Autodesk Inventor part; units mm, degrees
ref_plane "YZ Plane" through (0, 0, 0) normal (1, 0, 0) x (0, 1, 0)
ref_plane "XZ Plane" through (0, 0, 0) normal (0, 1, 0) x (-1, 0, 0)
ref_plane "XY Plane" through (0, 0, 0) normal (0, 0, 1) x (1, 0, 0)
sketch "Sketch1" plane through (0, 0, 0) normal (0, 0, 1) x (1, 0, 0)
  line L0 (0, -252.5291) -> (0, 252.5291) construction
  line L1 (-273, 0) -> (273, 0) construction
  line L2 (-195, 100) -> (195, 100)
  line L3 (195, 100) -> (195, -100)
  line L4 (195, -100) -> (-195, -100)
  line L5 (-195, -100) -> (-195, 100)
  line L6 (-178.1654, -28.1654) -> (-178.1654, 28.1654) construction
  line L7 (-178.1654, 28.1654) -> (178.1654, 28.1654) construction
  line L8 (178.1654, 28.1654) -> (178.1654, -28.1654) construction
  line L9 (178.1654, -28.1654) -> (-178.1654, -28.1654) construction
  circle A0 centre (0, 0) radius 180.3779 construction
  line L10 (-175, 25) -> (-175, -25) construction
  line L11 (-175, -25) -> (175, -25) construction
  line L12 (175, -25) -> (175, 25) construction
  line L13 (175, 25) -> (-175, 25) construction
  circle A1 centre (-175, 0) radius 6 construction
  point P0 (175, 0)
  point P1 (0, 25)
  point P2 (0, -25)
  dimension "d0" = 390
  dimension "d1" = 200
  dimension "d5" = 350
  dimension "d6" = 360.7559
  dimension "d14" = 350
  dimension "d15" = 12
  dimension "d54" = 353.5534
  dimension "d104" = 350
  dimension "d105" = 50
extrude "Extrusion1" add sketch "Sketch1" along normal blind 10
sketch "Sketch2" plane through (0, 0, 10) normal (0, 0, 1) x (1, 0, 0)
  point P0 (0, 0)
  point P1 (-175, -25)
  point P2 (-175, 25)
  point P3 (175, 25)
  point P4 (175, -25)
  point P5 (-175, 0)
  point P6 (175, 0)
  point P7 (0, 25)
  point P8 (0, -25)
hole "Hole1" at (-175, -25, 10) at (175, 25, 10) at (-175, 25, 10) at (175, -25, 10) at (0, 25, 10) at (0, -25, 10) direction (0, 0, -1) diameter 4.917 end through all
hole "Hole2" at (-175, 0, 10) at (175, 0, 10) direction (0, 0, -1) diameter 6.5 end through all counterbore diameter 16.5 counterbore depth 2
sketch "Sketch3" plane through (0, 0, 10) normal (0, 0, 1) x (1, 0, 0)
  line L0 (195, 100) -> (-195, 100) construction
  line L1 (-195, -100) -> (195, -100) construction
  line L2 (-195, 100) -> (-195, -100) construction
  line L3 (-273, 0) -> (273, 0) construction
  line L4 (0, -140) -> (0, 140) construction
  line L5 (195, -100) -> (195, 100) construction
  line L6 (-180, 90) -> (180, 90) construction
  line L7 (180, 90) -> (180, -90) construction
  line L8 (180, -90) -> (-180, -90) construction
  line L9 (-180, -90) -> (-180, 90) construction
  point P0 (0, 0)
  point P1 (-170, 80)
  point P2 (-150, 80)
  point P3 (-150, 80)
  point P4 (-130, 80)
  point P5 (-110, 80)
  point P6 (-90, 80)
  point P7 (-70, 80)
  point P8 (-50, 80)
  point P9 (-30, 80)
  point P10 (-10, 80)
  point P11 (10, 80)
  point P12 (30, 80)
  point P13 (50, 80)
  point P14 (70, 80)
  point P15 (90, 80)
  point P16 (110, 80)
  point P17 (130, 80)
  point P18 (150, 80)
  point P19 (170, 80)
  point P20 (-170, 60)
  point P21 (-150, 60)
  point P22 (-130, 60)
  point P23 (-110, 60)
  point P24 (-90, 60)
  point P25 (-70, 60)
  point P26 (-50, 60)
  point P27 (-30, 60)
  point P28 (-10, 60)
  point P29 (10, 60)
  point P30 (30, 60)
  point P31 (50, 60)
  point P32 (70, 60)
  point P33 (90, 60)
  point P34 (110, 60)
  point P35 (130, 60)
  point P36 (150, 60)
  point P37 (170, 60)
  point P38 (-170, 40)
  point P39 (-150, 40)
  point P40 (-130, 40)
  point P41 (-110, 40)
  point P42 (-90, 40)
  point P43 (-70, 40)
  point P44 (-50, 40)
  point P45 (-30, 40)
  point P46 (-10, 40)
  point P47 (10, 40)
  point P48 (30, 40)
  point P49 (50, 40)
  point P50 (70, 40)
  point P51 (90, 40)
  point P52 (110, 40)
  point P53 (130, 40)
  point P54 (150, 40)
  point P55 (170, 40)
  point P56 (-170, 20)
  point P57 (-150, 20)
  point P58 (-130, 20)
  point P59 (-110, 20)
  point P60 (-90, 20)
  point P61 (-70, 20)
  point P62 (-50, 20)
  point P63 (-30, 20)
  point P64 (-10, 20)
  point P65 (10, 20)
  point P66 (30, 20)
  point P67 (50, 20)
  point P68 (70, 20)
  point P69 (90, 20)
  point P70 (110, 20)
  point P71 (130, 20)
  point P72 (150, 20)
  point P73 (170, 20)
  point P74 (-170, 0)
  point P75 (-150, 0)
  point P76 (-130, 0)
  point P77 (-110, 0)
  point P78 (-90, 0)
  point P79 (-70, 0)
  point P80 (-50, 0)
  point P81 (-30, 0)
  point P82 (-10, 0)
  point P83 (10, 0)
  point P84 (30, 0)
  point P85 (50, 0)
  point P86 (70, 0)
  point P87 (90, 0)
  point P88 (110, 0)
  point P89 (130, 0)
  point P90 (150, 0)
  point P91 (170, 0)
  point P92 (-170, -20)
  point P93 (-150, -20)
  point P94 (-130, -20)
  point P95 (-110, -20)
  point P96 (-90, -20)
  point P97 (-70, -20)
  point P98 (-50, -20)
  point P99 (-30, -20)
  point P100 (-10, -20)
  point P101 (10, -20)
  point P102 (30, -20)
  point P103 (50, -20)
  point P104 (70, -20)
  point P105 (90, -20)
  point P106 (110, -20)
  point P107 (130, -20)
  point P108 (150, -20)
  point P109 (170, -20)
  point P110 (-170, -40)
  point P111 (-150, -40)
  point P112 (-130, -40)
  point P113 (-110, -40)
  point P114 (-90, -40)
  point P115 (-70, -40)
  point P116 (-50, -40)
  point P117 (-30, -40)
  point P118 (-10, -40)
  point P119 (10, -40)
  point P120 (30, -40)
  point P121 (50, -40)
  point P122 (70, -40)
  point P123 (90, -40)
  point P124 (110, -40)
  point P125 (130, -40)
  point P126 (150, -40)
  point P127 (170, -40)
  point P128 (-170, -60)
  point P129 (-150, -60)
  point P130 (-130, -60)
  point P131 (-110, -60)
  point P132 (-90, -60)
  point P133 (-70, -60)
  point P134 (-50, -60)
  point P135 (-30, -60)
  point P136 (-10, -60)
  point P137 (10, -60)
  point P138 (30, -60)
  point P139 (50, -60)
  point P140 (70, -60)
  point P141 (90, -60)
  point P142 (110, -60)
  point P143 (130, -60)
  point P144 (150, -60)
  point P145 (170, -60)
  point P146 (-170, -80)
  point P147 (-150, -80)
  point P148 (-130, -80)
  point P149 (-110, -80)
  point P150 (-90, -80)
  point P151 (-70, -80)
  point P152 (-50, -80)
  point P153 (-30, -80)
  point P154 (-10, -80)
  point P155 (10, -80)
  point P156 (30, -80)
  point P157 (50, -80)
  point P158 (70, -80)
  point P159 (90, -80)
  point P160 (110, -80)
  point P161 (130, -80)
  point P162 (150, -80)
  point P163 (170, -80)
  dimension "d25" = 10
  dimension "d26" = 360
  dimension "d27" = 180
  dimension "d28" = 10
  dimension "d29" = 10
  dimension "d30" = 20
  dimension "d33" = 20
  dimension "d36" = 20
  dimension "d39" = 15
hole "Hole3" [suppressed]
hole "Hole4" at (0, 0, 10) direction (0, 0, -1) diameter 11 end through all
sketch "Sketch4" plane through (0, 0, 0) normal (0, 0, -1) x (-1, 0, 0)
  circle A0 centre (175, 0) radius 3.25 construction
  circle A1 centre (-175, 0) radius 3.25 construction
  line L0 (195, -100) -> (-195, -100) construction
  line L1 (187.5, -100) -> (187.5, 100) construction
  line L2 (-195, 100) -> (195, 100) construction
  line L3 (273, 0) -> (-273, 0) construction
  line L4 (0, -140) -> (0, 140) construction
  line L5 (195, 100) -> (195, -100) construction
  point P0 (0, 0)
  point P1 (187.5, -90)
  point P2 (187.5, 90)
  point P3 (187.5, 0)
  point P4 (-187.5, -90)
  point P5 (-187.5, 90)
  point P6 (-187.5, 0)
  dimension "d62" = 180
  dimension "d63" = 7.5
hole "Hole5" at (-175, 0, 0) at (175, 0, 0) direction (0, 0, 1) diameter 6.5 end through all countersink diameter 14.5 countersink angle 90
hole "Hole6" at (-187.5, -90, 0) at (-187.5, 90, 0) at (-187.5, 0, 0) at (187.5, -90, 0) at (187.5, 0, 0) at (187.5, 90, 0) direction (0, 0, 1) diameter 3.242 end through all
sketch "Sketch10" plane through (-195, -100, 0) normal (0, -1, 0) x (1, 0, 0)
  line L0 (0, 0) -> (0, 10) construction
  line L1 (0, 6) -> (390, 6) construction
  line L2 (390, 0) -> (390, 10) construction
  line L3 (195, -2) -> (195, 12) construction
  line L4 (0, 10) -> (390, 10) construction
  line L5 (0, 0) -> (390, 0) construction
  point P0 (195, 0)
  point P1 (60, 6)
  point P2 (330, 6)
  dimension "d95" = 270
  dimension "d103" = 6
hole "Hole10" at (-135, -100, 6) at (135, -100, 6) direction (0, 1, 0) diameter 3.242 depth 15 tip angle 118
fillet "Fillet1" radius 2 4 edges at (-195, -100, 5) (195, -100, 5) (-195, 100, 5) (195, 100, 5)
properties part number "DLT-01-231B" material "Acrílico TP"
Source: CAD feature listing. Evaluate the final solid. Frame: model axes, mm. A direction names the side the tool comes from. Coordinates: 2 decimals unless noted, no trailing zeros. Answer as a JSON object with one key per item and string values.
Q1. Draft query along Y for faces 3 (the conical face through (-178.105, 1.615, 3.75)), 4 (the flat face through (-3, -21, 10)), 5 (the flat face through (3, -100, 5)). Return one class per face: released by +Y, released by -Y, zero draft, split by the parting line, or undercut.
Ans:
{"face 3": "undercut", "face 4": "zero draft", "face 5": "released by -Y"}
Q2. Set-up query: faces 1 (the cylindrical face through (166.82, 1.07, 8.99)), 2 (the conical face through (171.895, 1.615, 3.75)). Return all of +Z, -Z, +X, -X, +Y, -Y with unobstructed straight access to the full face (end or side cutting, diameter ignored); none if empty.
Ans:
{"face 1": "+Z", "face 2": "-Z"}
Q3. First-contact query: pin 1 Ø1.9 at (x, z) = (135, 6) entering from -Y; pin 2 Ø3 at (x, z) = (-135, 6) entering from -Y. Flat tips, straight axial feed; report the tip coordinate or a pass-through.
Ans:
{"pin 1": "stops at y = -84.6", "pin 2": "stops at y = -84.93"}
Q4. Material intervals for line 1 (X direction, y = 0, z = 7.5); line 2 (Y direction, x = 175, z = 5.6); line 3 (Y direction, x = 175, z = 9.5), sorted ascending. Write a range as [from, to].
Ans:
{"line 1": "x = [-195, -189.12], [-185.88, -178.25], [-171.75, -5.5], [5.5, 171.75], [178.25, 185.88], [189.12, 195]", "line 2": "y = [-100, -27.46], [-22.54, -3.25], [3.25, 22.54], [27.46, 100]", "line 3": "y = [-100, -27.46], [-22.54, -8.25], [8.25, 22.54], [27.46, 100]"}
